The listing builds one solid part. Answer for the finished solid, in the listing's coordinates (mm). A direction names the side the tool comes from. Coordinates: 2 decimals unless noted, no trailing zeros. Order: outer loops, then holes, each group sorted by start corner. A loop starts at its lowest first (then second) coordinate and runs counter-clockwise, first axis right, second up. Notation, with made-up numbers: (58.25, 81) -> (114.25, 81) arc R28 cw to (114.25, 107) -> close; hole circle Ø10 at (-27, 84.5). An arc over 180 degrees is marked (long way). Answer in a Markdown table with one row per item. Add a question column.
```python
from build123d import *

# Parameters (mm, degrees)
BOSS_EXTRUDE1_DEPTH = 3.048
SKETCH2_W           = 18.542
SKETCH2_H           = 2.8702
BOSS_EXTRUDE2_DEPTH = 3.048


with BuildPart() as part:
    # Sketch1 → Boss-Extrude1 (new body)
    with BuildSketch(Plane.XY):
        Polygon((-3.048, 12.0142), (0, 12.0142), (0, 19.6596), (2.54, 19.6596), (2.54, 6.2738), (18.542, 6.2738), (18.542, 22.5298), (21.4122, 22.5298), (21.4122, 6.7818), (36.9062, 6.7818), (36.9062, 22.5298), (39.3446, 22.5298), (39.3446, 6.7818), (54.8386, 6.7818), (54.8386, 22.5298), (56.134, 22.5298), (56.134, 12.0142), (59.182, 12.0142), (59.182, 4.7244), (52.324, 4.7244), (52.324, 1.5494), (3.81, 1.5494), (3.81, 4.7244), (-3.048, 4.7244), align=None)
    extrude(amount=BOSS_EXTRUDE1_DEPTH)

    # Sketch2 → Boss-Extrude2 (add)
    with BuildSketch(Plane.XY.offset(3.048)):
        with Locations((9.271, 21.0947)):
            Rectangle(SKETCH2_W, SKETCH2_H)
    extrude(amount=-BOSS_EXTRUDE2_DEPTH)


solid = part.part
```
Q1. Determine the mould class of faces 5 (the face through (28, 1.549, 2)), 6 (the face through (-2, 12.014, 2)), 7 (the face through (18.542, 13, 2)) for opening direction Y: +Y half, -Y half, draft (parallel to the pull), parting line (faces both ways), or undercut.
Q2. A cutting plane is placed at C-C (z = 0.95). Determine the outline of the cut face in (x, y).
Q3. A cutting plane is placed at B-B (x = 15). Determine the outline of the cut face in (y, z).
Q4. Given pin 1 (0.9 mm diameter, centred on y = 16, z = 1.5, fed in from +X); pin 2 (2 mm diameter, centred on x = 35, y = 14, fed in from -Z); pin 3 (1.5 mm diameter, centred on x = 30, z = 0.5, fed in from +Y), each flat-ended and moving along its own axis, determine where each tip first touches the part or whether it passes through.
Q5. Straight lines are drawn through the part: line 1 (X direction, y = 10, z = 1.2); line 2 (X direction, y = 19.5, z = 2); line 3 (X direction, y = 21.75, z = 1.4). For each, find the intervals that lie inside material, in ascending order.
Q6. For faces 1 (the face through (47, 6.782, 2)), 2 (the face through (58, 12.014, 2)), 3 (the face through (56, 4.724, 2)), 4 (the face through (10, 6.274, 2)), determine the directions among +Z, -Z, +X, -X, +Y, -Y from which every point of the face is accessible in a straight line to the end or side of a thin tool.
Q7. A cutting plane is placed at D-D (y = 13.25). Determine the outline of the cut face in (x, z), then the cut area to 3 significant figures.
Q8. A cutting plane is placed at A-A (y = 10.75). Determine the outline of the cut face in (x, z), then the cut area to 3 significant figures.
Returned:
| question | item | result |
|---|---|---|
| 1 | face 5 | -Y half |
| 1 | face 6 | +Y half |
| 1 | face 7 | undercut |
| 2 | outline | (-3.05, 4.72) -> (3.81, 4.72) -> (3.81, 1.55) -> (52.32, 1.55) -> (52.32, 4.72) -> (59.18, 4.72) -> (59.18, 12.01) -> (56.13, 12.01) -> (56.13, 22.53) -> (54.84, 22.53) -> (54.84, 6.78) -> (39.34, 6.78) -> (39.34, 22.53) -> (36.91, 22.53) -> (36.91, 6.78) -> (21.41, 6.78) -> (21.41, 22.53) -> (0, 22.53) -> (0, 12.01) -> (-3.05, 12.01) -> close; hole (2.54, 6.27) -> (18.54, 6.27) -> (18.54, 19.66) -> (2.54, 19.66) -> close |
| 3 | outline | (1.55, 0) -> (6.27, 0) -> (6.27, 3.05) -> (1.55, 3.05) -> close; (19.66, 0) -> (22.53, 0) -> (22.53, 3.05) -> (19.66, 3.05) -> close |
| 4 | pin 1 | stops at x = 56.13 |
| 4 | pin 2 | passes through |
| 4 | pin 3 | stops at y = 6.78 |
| 5 | line 1 | x = -3.05 to 2.54, 18.54 to 21.41, 36.91 to 39.34, 54.84 to 59.18 |
| 5 | line 2 | x = 0 to 2.54, 18.54 to 21.41, 36.91 to 39.34, 54.84 to 56.13 |
| 5 | line 3 | x = 0 to 21.41, 36.91 to 39.34, 54.84 to 56.13 |
| 6 | face 1 | +Z, -Z, +Y |
| 6 | face 2 | +Z, -Z, +X, +Y |
| 6 | face 3 | +Z, -Z, +X, -Y |
| 6 | face 4 | +Z, -Z |
| 7 | outline | (0, 0) -> (2.54, 0) -> (2.54, 3.05) -> (0, 3.05) -> close; (18.54, 0) -> (21.41, 0) -> (21.41, 3.05) -> (18.54, 3.05) -> close; (36.91, 0) -> (39.34, 0) -> (39.34, 3.05) -> (36.91, 3.05) -> close; (54.84, 0) -> (56.13, 0) -> (56.13, 3.05) -> (54.84, 3.05) -> close |
| 7 | area | 27.9 mm² |
| 8 | outline | (-3.05, 0) -> (2.54, 0) -> (2.54, 3.05) -> (-3.05, 3.05) -> close; (18.54, 0) -> (21.41, 0) -> (21.41, 3.05) -> (18.54, 3.05) -> close; (36.91, 0) -> (39.34, 0) -> (39.34, 3.05) -> (36.91, 3.05) -> close; (54.84, 0) -> (59.18, 0) -> (59.18, 3.05) -> (54.84, 3.05) -> close |
| 8 | area | 46.5 mm² |
